Design review of the part built by this model. Coordinates are the model's own, in mm. Give positions to 0.01 mm unless a question says otherwise; leave off trailing zeros.
```python
from build123d import *

# Parameters (mm, degrees)
ESQUISSE1_R             = 1
ESQUISSE1_W             = 27
ESQUISSE1_H             = 19.5
ESQUISSE1_W_2           = 5
ESQUISSE1_H_2           = 14
BOSS_EXTRU_1_DEPTH      = 2
ENL_V_START             = -1
ENL_V_MAT_EXTRU_1_DEPTH = 1
CONG_1_R                = 0.5


with BuildPart() as part:
    # Esquisse1 → Boss.-Extru.1 (new body)
    with BuildSketch(Plane.XY):
        with BuildLine():
            Line((33, 30), (-33, 30))
            ThreePointArc((-33, 30), (-37.949747468, 27.949747468), (-40, 23))
            Line((-40, 23), (-40, -23))
            ThreePointArc((-40, -23), (-37.949747468, -27.949747468), (-33, -30))
            Line((-33, -30), (33, -30))
            ThreePointArc((33, -30), (37.949747468, -27.949747468), (40, -23))
            Line((40, -23), (40, 23))
            ThreePointArc((40, 23), (37.949747468, 27.949747468), (33, 30))
        make_face()
        with Locations((-32, 12.05)):
            Circle(ESQUISSE1_R, mode=Mode.SUBTRACT)
        with Locations((-7, 12.05)):
            Circle(ESQUISSE1_R, mode=Mode.SUBTRACT)
        with Locations((-7, -12.25)):
            Circle(ESQUISSE1_R, mode=Mode.SUBTRACT)
        with Locations((-32, -12.25)):
            Circle(ESQUISSE1_R, mode=Mode.SUBTRACT)
        with Locations((8, 4.2)):
            Circle(ESQUISSE1_R, mode=Mode.SUBTRACT)
        with Locations((8, -4.2)):
            Circle(ESQUISSE1_R, mode=Mode.SUBTRACT)
        with Locations((-19.5, 0)):
            Rectangle(ESQUISSE1_W, ESQUISSE1_H, mode=Mode.SUBTRACT)
        with Locations((21.5, 0)):
            Rectangle(ESQUISSE1_W_2, ESQUISSE1_H_2, mode=Mode.SUBTRACT)
    extrude(amount=BOSS_EXTRU_1_DEPTH)

    # Esquisse2 → Enlèv. mat.-Extru.1 (cut)
    with BuildSketch(Plane.XY.offset(2).offset(ENL_V_START)):
        with BuildLine():
            Line((40, -23), (40, 23))
            ThreePointArc((40, 23), (37.949747468, 27.949747468), (33, 30))
            Line((33, 30), (-33, 30))
            ThreePointArc((-33, 30), (-37.949747468, 27.949747468), (-40, 23))
            Line((-40, 23), (-40, -23))
            ThreePointArc((-40, -23), (-37.949747468, -27.949747468), (-33, -30))
            Line((-33, -30), (33, -30))
            ThreePointArc((33, -30), (37.949747468, -27.949747468), (40, -23))
        make_face()
        with BuildLine():
            Line((38, -23), (38, 23))
            ThreePointArc((38, 23), (36.535533906, 26.535533906), (33, 28))
            Line((33, 28), (-33, 28))
            ThreePointArc((-33, 28), (-36.535533906, 26.535533906), (-38, 23))
            Line((-38, 23), (-38, -23))
            ThreePointArc((-38, -23), (-36.535533906, -26.535533906), (-33, -28))
            Line((-33, -28), (33, -28))
            ThreePointArc((33, -28), (36.535533906, -26.535533906), (38, -23))
        make_face(mode=Mode.SUBTRACT)
    extrude(amount=ENL_V_MAT_EXTRU_1_DEPTH, mode=Mode.SUBTRACT)

    # Congé1
    cong_1_edges = [part.edges().sort_by_distance(p)[0] for p in [
        (37.949747468, 27.949747468, 0),
        (40, 0, 0),
        (37.949747468, -27.949747468, 0),
        (0, -30, 0),
        (-37.949747468, -27.949747468, 0),
        (-40, 0, 0),
        (-37.949747468, 27.949747468, 0),
        (37.949747468, 27.949747468, 1),
        (40, 0, 1),
        (37.949747468, -27.949747468, 1),
        (0, -30, 1),
        (-37.949747468, -27.949747468, 1),
        (-40, 0, 1),
        (-37.949747468, 27.949747468, 1),
        (36.535533906, 26.535533906, 2),
        (38, 0, 2),
        (36.535533906, -26.535533906, 2),
        (0, -28, 2),
        (-36.535533906, -26.535533906, 2),
        (-38, 0, 2),
        (-36.535533906, 26.535533906, 2),
        (36.535533906, 26.535533906, 1),
        (38, 0, 1),
        (36.535533906, -26.535533906, 1),
        (0, -28, 1),
        (-36.535533906, -26.535533906, 1),
        (-38, 0, 1),
        (-36.535533906, 26.535533906, 1),
        (0, 30, 0),
        (0, 30, 1),
        (0, 28, 2),
        (0, 28, 1),
    ]]
    fillet(cong_1_edges, radius=CONG_1_R - 0.0001)  # a hair under: the kernel refuses the full size


solid = part.part
```
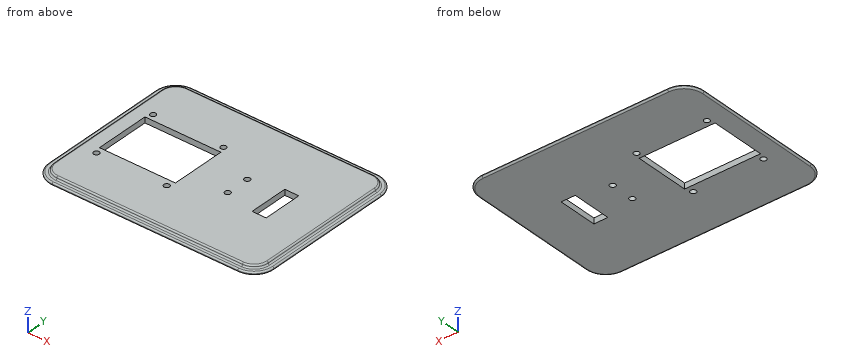
(1) Consider section A-A, the plane y = -12.25. Give the number of separate pieces and of enclosed holes in the cut face, then the cut area to 3 significant figures.
Resolved:
separate pieces: 3
enclosed holes: 0
area: 148 mm2
(2) Clearance check with a flat-ended pin moving along its axis: P1, Ø0.6, axis at y = 1.5, z = 1, coming from the +X side. State where the tip first meets the part, or that it passes through.
Resolved:
P1: stops at x = 39.96
(3) To check wall thickness, follow L1, parallel to X at y = -4, z = 1.6; L2, parallel to Y at x = -7, z = 1.4; L3, parallel to Y at x = 8, z = 0.4. State the ranges of each line that lie inside material, in increasing order.
Resolved:
L1: x = -37.99 to -33, -6 to 7.02, 8.98 to 19, 24 to 37.99
L2: y = -28.01 to -13.25, -11.25 to -9.75, 9.75 to 11.05, 13.05 to 28.01
L3: y = -29.99 to -5.2, -3.2 to 3.2, 5.2 to 29.99
